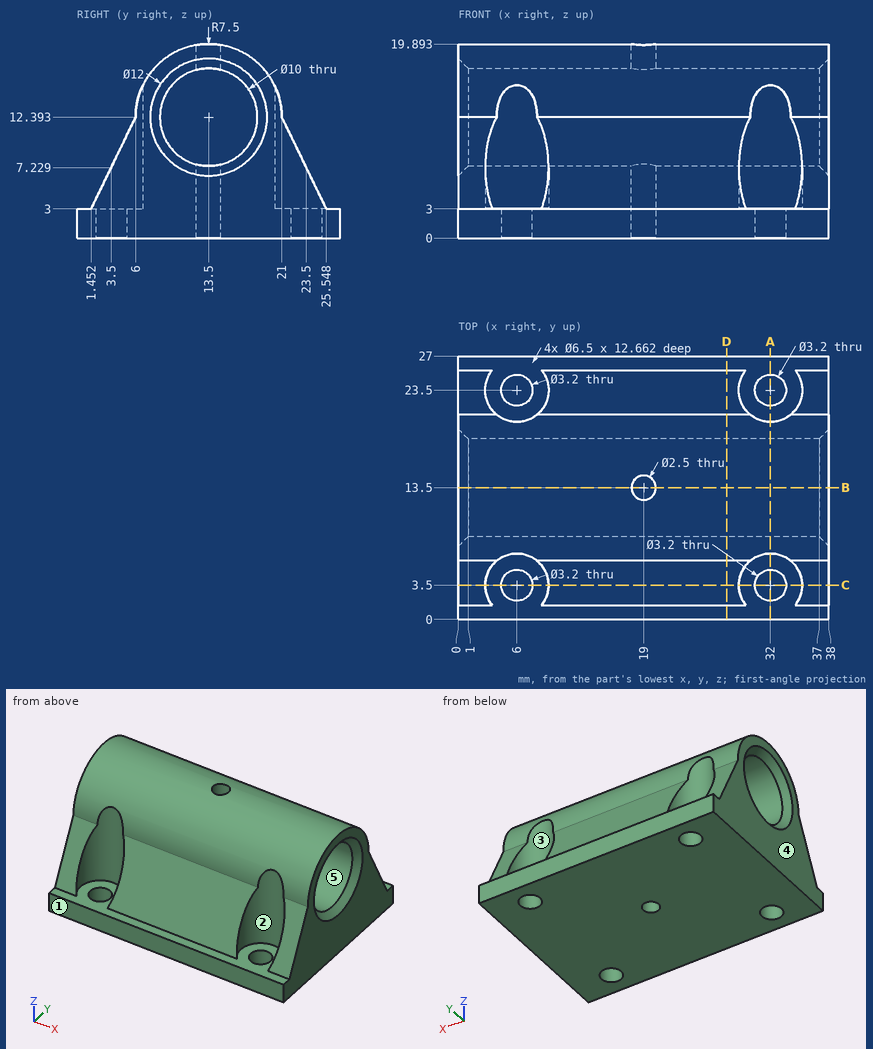
Geometry check sheet. Reference: drawing and pictorial views, mm from the part's lowest x, y, z. A direction names the side the tool comes from. Round coordinates to 2 decimals unless told otherwise and drop trailing zeros. Loops run counter-clockwise (first coordinate to the right, second up) from the corner with the lowest first, then second, coordinate; pieces in that order, holes last. Notation, with made-up numbers: (3.5, 77) -> (7.5, 77) arc R22 cw to (7.5, 86) -> close; hole circle Ø1 at (44, 38.5). An arc over 180 degrees is marked (long way). Answer as a JSON object with one key per item and string values. Group by question number.
Item 1: Depth check by flat-ended pin: pin 1 Ø4 at (x, y) = (6, 3.5) entering from +Z; pin 2 Ø5 at (x, z) = (32.5, 14) entering from +Y; pin 3 Ø3.5 at (x, y) = (11, 23) entering from +Z (1 decimal). Enter the tip coordinate at first touch or a pass-through.
Item 2: Cross-section at D-D, the plane x = 27.5. Record the cut outline in (y, z).
Item 3: Thickness scan on line 1 along X through (y, z) = (3.5, 1.6); line 2 along Y through (x, z) = (6, 2.2); line 3 along X through (y, z) = (13.5, 3). Record the ranges inside material, lowest first.
Item 4: Cross-section at A-A, the plane x = 32. Record the cut outline in (y, z), plus the area to 3 significant figures.
Item 5: Release check for a two-part mould opening along X. For the marked faces 3, 4 and 5 record: pulls with the +X half, pulls with the -X half, needs draft (parallel to the pull), parting line crosses it, or undercut.
Item 6: Cross-section at B-B, the plane y = 13.5. Record the cut outline in (x, z), plus the area to 3 significant figures.
Item 7: Cross-section at C-C, the plane y = 3.5. Record the cut outline in (x, z).
Item 8: Set-up check for the marked faces 1 and 2: record each of +Z, -Z, +X, -X, +Y, -Y from which the full face is reachable in a straight line by a thin tool's end or side.
Determined:
{
 "1": {"pin 1": "stops at z = 3", "pin 2": "stops at y = 21.11", "pin 3": "stops at z = 11.9"},
 "2": {"outline": "(0, 0) -> (27, 0) -> (27, 3) -> (25.55, 3) -> (21, 12.39) arc R7.5 ccw to (6, 12.39) -> (1.45, 3) -> (0, 3) -> close; hole circle Ø10 at (13.5, 12.39)"},
 "3": {"line 1": "x = 0 to 4.4, 7.6 to 30.4, 33.6 to 38", "line 2": "y = 0 to 1.9, 5.1 to 21.9, 25.1 to 27", "line 3": "x = 0 to 17.75, 20.25 to 38"},
 "4": {"outline": "(0, 0) -> (1.9, 0) -> (1.9, 3) -> (0, 3) -> close; (5.1, 0) -> (21.9, 0) -> (21.9, 3) -> (20.25, 3) -> (20.25, 15.66) arc R7.5 ccw to (6.75, 15.66) -> (6.75, 3) -> (5.1, 3) -> close; (25.1, 0) -> (27, 0) -> (27, 3) -> (25.1, 3) -> close; hole circle Ø10 at (13.5, 12.39)", "area": "195 mm²"},
 "5": {"face 3": "undercut", "face 4": "pulls with the -X half", "face 5": "needs draft"},
 "6": {"outline": "(0, 0) -> (17.75, 0) -> (17.75, 7.39) -> (1, 7.39) -> (0, 6.39) -> close; (0, 18.39) -> (1, 17.39) -> (17.75, 17.39) -> (17.75, 19.89) -> (0, 19.89) -> close; (20.25, 0) -> (38, 0) -> (38, 6.39) -> (37, 7.39) -> (20.25, 7.39) -> close; (20.25, 17.39) -> (37, 17.39) -> (38, 18.39) -> (38, 19.89) -> (20.25, 19.89) -> close", "area": "349 mm²"},
 "7": {"outline": "(0, 0) -> (4.4, 0) -> (4.4, 3) -> (2.75, 3) -> (2.75, 7.23) -> (0, 7.23) -> close; (7.6, 0) -> (30.4, 0) -> (30.4, 3) -> (28.75, 3) -> (28.75, 7.23) -> (9.25, 7.23) -> (9.25, 3) -> (7.6, 3) -> close; (33.6, 0) -> (38, 0) -> (38, 7.23) -> (35.25, 7.23) -> (35.25, 3) -> (33.6, 3) -> close"},
 "8": {"face 1": "+Z, -Z, +X, -X, -Y", "face 2": "+Z"}
}
